Input: dimensioned drawing with shaded views. Units: mm. Origin: part minimum x, y, z. Coordinates: 2 decimals unless noted, no trailing zeros. Loops run counter-clockwise (first coordinate to the right, second up) from the corner with the lowest first, then second, coordinate; pieces in that order, holes last. Notation, with made-up numbers: M -22,-11 L 37,-11 A12 cw 37,4 Z; hole C -22,-21 d11. An arc over 180 degrees is marked long. Write item = value, one per line. Start each with the question number.
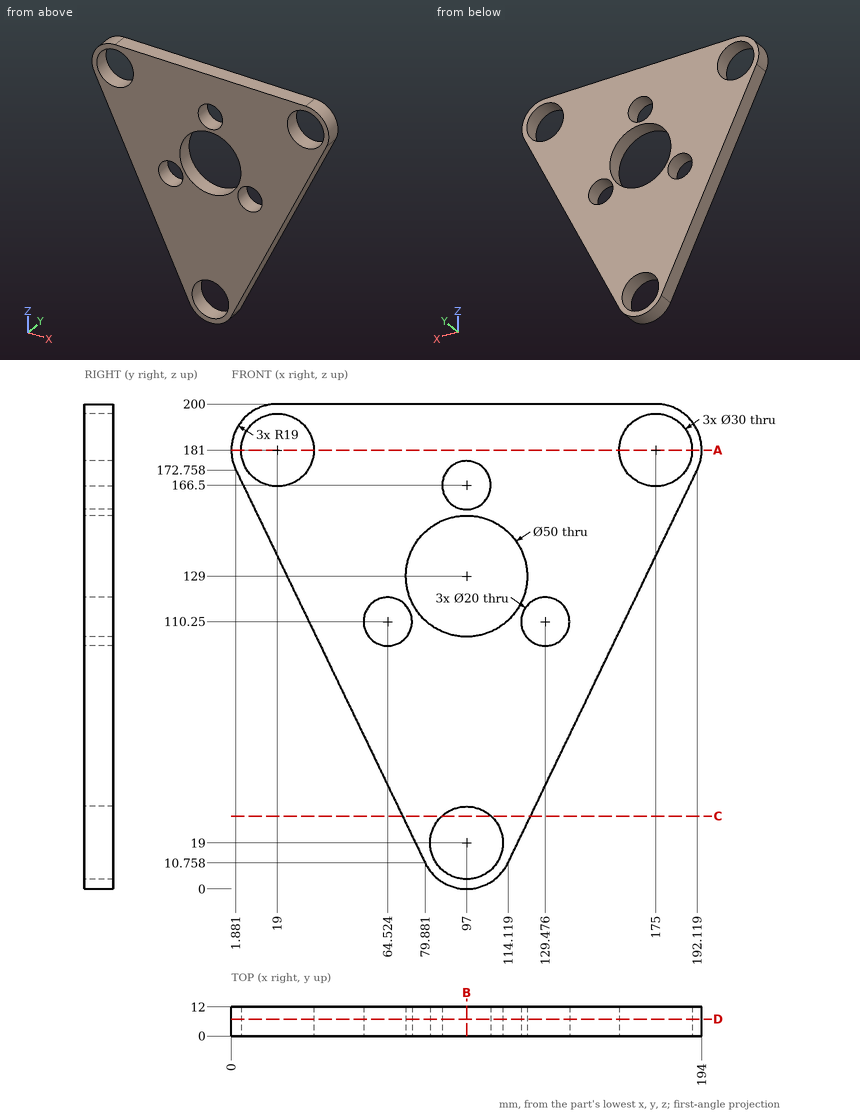
Item 1: First-contact query: pin 1 (3 mm diameter, centred on y = 3, z = 128.5, fed in from -X); pin 2 (1 mm diameter, centred on x = 131.5, y = 10.5, fed in from -Z) (1 decimal); pin 3 (3 mm diameter, centred on x = 52, y = 8, fed in from -Z). Flat tips, straight axial feed; report the tip coordinate or a pass-through.
Item 2: Section query C-C (z = 30). Return the cut outline in (x, y).
Item 3: Line query: line 1 (X direction, y = 5.75, z = 181); line 2 (X direction, y = 10, z = 172.5) (1 decimal); line 3 (Z direction, x = 165, y = 2) (1 decimal). Output: solid intervals per line, ascending. Write a range as from..to.
Item 4: Section query A-A (z = 181). Return the cut outline in (x, y), plus the area to 3 significant figures.
Item 5: Section query B-B (x = 97). Return the cut outline in (y, z).
Item 6: Section query D-D (y = 7). Count the separate pieces of the cut face and the enclosed holes in it, plus the area to 3 significant figures.
Verdict:
q1.pin_1 = 22.47
q1.pin_2 = 45.8
q1.pin_3 = 65.55
q2.outline = M 70.62,0 L 86.8,0 L 86.8,12 L 70.62,12 Z; M 107.2,0 L 123.38,0 L 123.38,12 L 107.2,12 Z
q3.line_1 = 0..4, 34..160, 190..194
q3.line_2 = 2..6.6, 31.4..89, 105..162.6, 187.4..192
q3.line_3 = 116.4..169.8, 192.2..200
q4.outline = M 0,0 L 4,0 L 4,12 L 0,12 Z; M 34,0 L 160,0 L 160,12 L 34,12 Z; M 190,0 L 194,0 L 194,12 L 190,12 Z
q4.area = 1,610 mm2
q5.outline = M 0,0 L 12,0 L 12,4 L 0,4 Z; M 0,34 L 12,34 L 12,104 L 0,104 Z; M 0,154 L 12,154 L 12,156.5 L 0,156.5 Z; M 0,176.5 L 12,176.5 L 12,200 L 0,200 Z
q6.separate_pieces = 1
q6.enclosed_holes = 7
q6.area = 18,500 mm2
